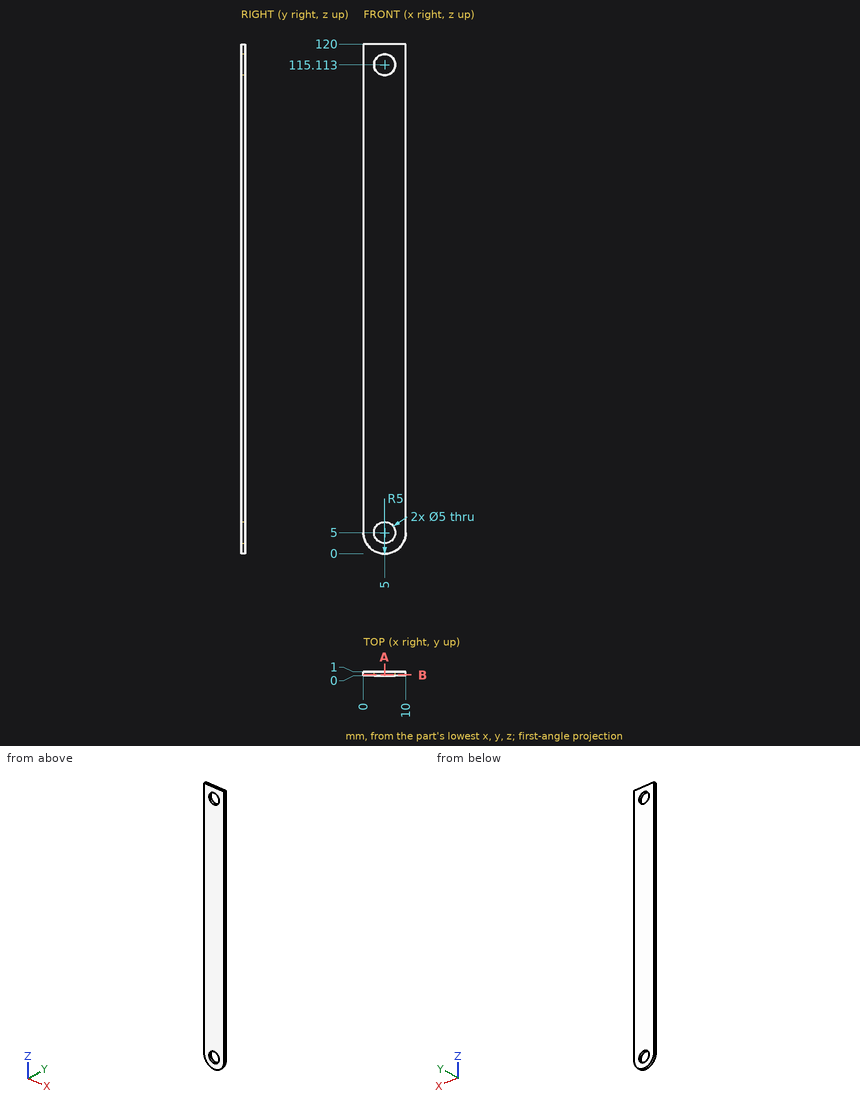
The drawing under review shows one solid part. Ordinate dimensions are in mm from its lowest x, y, z. Coordinates: 2 decimals unless noted, no trailing zeros. Write each loop counter-clockwise with the first axis right and the second up, starting at its lowest first coordinate (ties: lowest second). Pieces come first, ordered by that corner, then holes. Notation, with made-up numbers: (-21, 61) - (-9, 61) arc R24 ccw to (-9, 100) - close; hole circle Ø10 at (-29, 82.5). An arc over 180 degrees is marked (long way). Answer in a Markdown table with one row per item. Add a question column.
Q1. We need section B-B, the plane y = 0.25. State the section outline as (x, z) points, and give its area (3 significant figures).
Q2. For probe 1 along Z at (x, y) = (4.75, 0.9); probe 2 along Z at (x, y) = (7.25, 0.5); probe 3 along X at (y, z) = (0.25, 5), list the stretches that pass through material, from the lowest coordinate up.
Q3. For P1, Ø3, axis at x = 5, z = 115.113, coming from the +Y side, flat-tipped, find the tip position at first contact; note if it passes through.
Q4. We need section A-A, the plane x = 5. State the section outline as (y, z) points, and give its area (3 significant figures).
Answer list:
| question | item | result |
|---|---|---|
| 1 | outline | (0, 5) arc R5 ccw to (10, 5) - (10, 120) - (0, 120) - close; hole circle Ø5 at (5, 5); hole circle Ø5 at (5, 115.11) |
| 1 | area | 1,150 mm2 |
| 2 | probe 1 | z = 0.01 to 2.51, 7.49 to 112.63, 117.6 to 120 |
| 2 | probe 2 | z = 0.53 to 3.91, 6.09 to 114.02, 116.2 to 120 |
| 2 | probe 3 | x = 0 to 2.5, 7.5 to 10 |
| 3 | P1 | passes through |
| 4 | outline | (0, 0) - (1, 0) - (1, 2.5) - (0, 2.5) - close; (0, 7.5) - (1, 7.5) - (1, 112.61) - (0, 112.61) - close; (0, 117.61) - (1, 117.61) - (1, 120) - (0, 120) - close |
| 4 | area | 110 mm2 |
